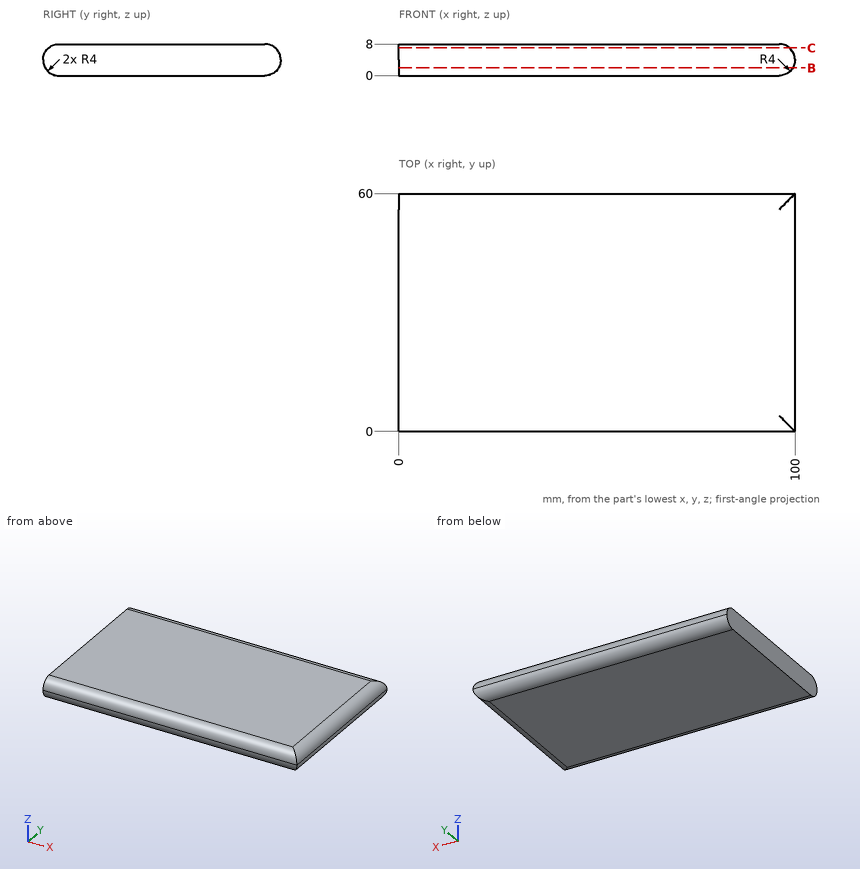
Here's the drawing with two shaded views (mm, measured from the low corner). I have some questions. Give positions to 0.01 mm unless a question says otherwise; leave off trailing zeros. Write each loop counter-clockwise with the first axis right and the second up, starting at its lowest first coordinate (ties: lowest second). Pieces come first, ordered by that corner, then holes. Notation, with made-up numbers: (58.25, 29) -> (68.25, 29) arc R34 ccw to (68.25, 62) -> close; hole circle Ø2 at (-34, 49). An arc over 180 degrees is marked (long way). Answer as a JSON object with one key per item and string values. Group by question number.
Item 1: I'm going to push a flat-ended pin straight in: P1, Ø1, axis at y = 31.5, z = 1, coming from the +X side. Where does the tip first touch, or does it pass through?
Item 2: Suppose I cut it at C-C (z = 7). Please give me the cut outline in (x, y), plus the area to 3 significant figures.
Item 3: Please list where these lines run through material, in increasing order: line 1 (X direction, y = 25, z = 1); line 2 (X direction, y = 35.5, z = 6); line 3 (Y direction, x = 96.5, z = 7). Write a range as [from, to].
Item 4: Suppose I cut it at B-B (z = 2). Please give me the cut outline in (x, y), plus the area to 3 significant figures.
Findings:
{
 "1": {"P1": "stops at x = 99.12"},
 "2": {"outline": "(0, 1.35) -> (98.65, 1.35) -> (98.65, 58.65) -> (0, 58.65) -> close", "area": "5,650 mm²"},
 "3": {"line 1": "x = [0, 98.65]", "line 2": "x = [0, 99.46]", "line 3": "y = [1.35, 58.65]"},
 "4": {"outline": "(0, 0.54) -> (99.46, 0.54) -> (99.46, 59.46) -> (0, 59.46) -> close", "area": "5,860 mm²"}
}
